Read the model definition and answer for the solid it produces. Units are mm, in the model's axes. A direction names the side the tool comes from. Coordinates: 2 decimals unless noted, no trailing zeros. Write each loop counter-clockwise with the first axis right and the second up, starting at its lowest first coordinate (ties: lowest second). Pieces come first, ordered by that corner, then holes. Notation, with made-up numbers: (21, 26.25) -> (26, 26.25) arc R32 cw to (26, 59.25) -> close; hole circle Ø2 at (-2.75, 87). An arc over 180 degrees is marked (long way). Write item = value, one per line. Start each with the question number.
1) Section D-D (y = -38.5) is taken. Determine the outline of the cut face in (x, z).
2) Find the intervals of material crossed by line 1 along Z through (x, y) = (37, -33); line 2 along X through (y, z) = (-38.5, 36), in increasing order. Write a range as from..to.
3) Section B-B (x = 21.15) is taken. Determine the outline of the cut face in (y, z).
4) Flat-ended cylindrical pins translate along their axes: pin 1 Ø1.5 at (x, z) = (38, 42) entering from +Y; pin 2 Ø2 at (x, y) = (5, -28.5) entering from +Z. Find the tip coordinate at first contact, or state that the pin passes through.
5) Section A-A (z = 15.5) is taken. Determine the outline of the cut face in (x, y).
6) Section C-C (y = -3.5) is taken. Determine the outline of the cut face in (x, z).
7) A tool of negligible diameter and unlimited length cuts with its end or side. For faces 1 (the face through (30, -30, 48)), 2 (the face through (39.8, -39.8, 23.7)), from which of +Z, -Z, +X, -X, +Y, -Y can it reach the whole face along a straight path? Write none if from no direction.
from build123d import *

# Parameters (mm, degrees)
SKETCH1_W           = 42.3
SKETCH1_H           = 42.3
BOSS_EXTRUDE1_DEPTH = 48
SKETCH2_R           = 11
BOSS_EXTRUDE2_DEPTH = 2
CHAMFER1_SIZE       = 5


with BuildPart() as part:
    # Sketch1 → Boss-Extrude1 (new body)
    with BuildSketch(Plane.XY):
        with Locations((21.15, -21.15)):
            Rectangle(SKETCH1_W, SKETCH1_H)
    extrude(amount=BOSS_EXTRUDE1_DEPTH)

    # Sketch2 → Boss-Extrude2 (add)
    with BuildSketch(Plane.XY.offset(48)):
        with Locations((21.15, -21.15)):
            Circle(SKETCH2_R)
    extrude(amount=BOSS_EXTRUDE2_DEPTH)

    # Chamfer1
    chamfer1_edges = [part.edges().sort_by_distance(p)[0] for p in [
        (0, 0, 24),
        (42.3, 0, 24),
        (42.3, -42.3, 24),
        (0, -42.3, 24),
    ]]
    chamfer(chamfer1_edges, length=CHAMFER1_SIZE)


solid = part.part
Answer key:
q1.outline = (1.2, 0) -> (41.1, 0) -> (41.1, 48) -> (1.2, 48) -> close
q2.line_1 = 0..48
q2.line_2 = 1.2..41.1
q3.outline = (-42.3, 0) -> (0, 0) -> (0, 48) -> (-10.15, 48) -> (-10.15, 50) -> (-32.15, 50) -> (-32.15, 48) -> (-42.3, 48) -> close
q4.pin_1 = 0
q4.pin_2 = 48
q5.outline = (0, -37.3) -> (5, -42.3) -> (37.3, -42.3) -> (42.3, -37.3) -> (42.3, -5) -> (37.3, 0) -> (5, 0) -> (0, -5) -> close
q6.outline = (1.5, 0) -> (40.8, 0) -> (40.8, 48) -> (1.5, 48) -> close
q7.face_1 = +Z
q7.face_2 = +Z, -Z, +X, -Y
